Autodesk Inventor part; units mm, degrees
ref_plane "YZ Plane" through (0, 0, 0) normal (1, 0, 0) x (0, 1, 0)
ref_plane "XZ Plane" through (0, 0, 0) normal (0, 1, 0) x (-1, 0, 0)
ref_plane "XY Plane" through (0, 0, 0) normal (0, 0, 1) x (1, 0, 0)
sketch "Sketch1" plane through (0, 0, 0) normal (0, 1, 0) x (-1, 0, 0)
  line L0 (-4.5005, -6.5) -> (-3.283, -6.5)
  line L1 (-3.283, -6.5) -> (-2.9693, -6.948)
  line L2 (-2.9693, -6.948) -> (-2.9693, -8.2299)
  line L3 (-2.9693, -8.2299) -> (-2.0718, -8.2299)
  line L4 (-2.0718, -8.2299) -> (-2.0718, -7.0351)
  line L5 (-2.0718, -7.0351) -> (-1.8086, -6.5)
  line L6 (-1.8086, -6.5) -> (-0.6909, -6.5)
  line L7 (-0.6909, -6.5) -> (-0.4278, -7.0351)
  line L8 (-0.4278, -7.0351) -> (-0.4278, -8.2299)
  line L9 (-0.4278, -8.2299) -> (0.4698, -8.2299)
  line L10 (0.4698, -8.2299) -> (0.4698, -6.948)
  line L11 (0.4698, -6.948) -> (0.7835, -6.5)
  line L12 (0.7835, -6.5) -> (1.8077, -6.5)
  line L13 (1.8077, -6.5) -> (2.0708, -7.0351)
  line L14 (2.0708, -7.0351) -> (2.0708, -8.2299)
  line L15 (2.0708, -8.2299) -> (2.9683, -8.2299)
  line L16 (2.9683, -8.2299) -> (2.9683, -6.948)
  line L17 (2.9683, -6.948) -> (3.2821, -6.5)
  line L18 (3.2821, -6.5) -> (4.4995, -6.5)
  line L19 (4.4995, -6.5) -> (5.4995, -5.5)
  line L20 (5.4995, -5.5) -> (5.4995, 1.9247)
  line L21 (5.4995, 1.9247) -> (2.4995, 5.5)
  line L22 (2.4995, 5.5) -> (0.4698, 5.5)
  line L23 (0.4698, 5.5) -> (0.4698, 6.6191)
  line L24 (0.4698, 6.6191) -> (-0.4278, 6.6191)
  line L25 (-0.4278, 6.6191) -> (-0.4278, 5.5)
  line L26 (-0.4278, 5.5) -> (-2.5005, 5.5)
  line L27 (-2.5005, 5.5) -> (-5.5005, 1.9247)
  line L28 (-5.5005, 1.9247) -> (-5.5005, -5.5)
  line L29 (-5.5005, -5.5) -> (-4.5005, -6.5)
  circle A0 centre (-0.0005, -2.3274) radius 0.7145
  line L30 (6.998, 7.6726) -> (-7.002, 7.6726)
  line L31 (-7.002, 7.6726) -> (-7.002, -17.3274)
  line L32 (-7.002, -17.3274) -> (6.998, -17.3274)
  line L33 (6.998, -17.3274) -> (6.998, 7.6726)
  circle A1 centre (-0.0005, -2.3274) radius 2.75
  line L34 (-0.002, -21.2436) -> (-0.002, 13.4129) construction
  point P0 (-0.002, -0.846)
  dimension "d0" = 14
  dimension "d1" = 25
  dimension "d2" = 5.5
  dimension "d19" = 7
  dimension "d22" = 10
extrude "Extrusion1" add sketch "Sketch1" along normal blind 1.6 contours L29 L28 L27 L26 L25 L24 L23 L22 L21 L20 L19 L18 L17 L16 L15 L14 L13 L12 L11 L10 L9 L8 L7 L6 L5 L4 L3 L2 L1 L0 | L33 L32 L31 L30
sketch "Sketch2" plane through (0, 1.6, 0) normal (0, 1, 0) x (1, 0, 0)
  line L0 (-6.998, 17.3274) -> (-6.998, -7.6726)
  line L1 (7.002, 17.3274) -> (-6.998, 17.3274)
  line L2 (-6.998, -7.6726) -> (7.002, -7.6726)
  line L3 (7.002, -7.6726) -> (7.002, 17.3274)
  line L4 (7.002, 17.3274) -> (-6.998, 17.3274)
  line L5 (-6.998, 17.3274) -> (-6.998, -7.6726)
  circle A0 centre (5.002, -4.6726) radius 0.8
  circle A1 centre (5.002, 11.3274) radius 0.8
  circle A2 centre (-4.998, 11.3274) radius 0.8
  circle A3 centre (-4.998, -4.6726) radius 0.8
  point P0 (0, 0)
  dimension "d5" = 1.6
  dimension "d6" = 1.6
  dimension "d7" = 1.6
  dimension "d8" = 1.6
  dimension "d9" = 2
  dimension "d10" = 3
  dimension "d11" = 3
  dimension "d12" = 2
  dimension "d13" = 2
  dimension "d15" = 2
  dimension "d20" = 16
  dimension "d21" = 16
extrude "Extrusion2" cut sketch "Sketch2" against normal blind 1.6 contours A0 | A1 | A2 | A3
fillet "Fillet1" radius 2 4 edges at (-6.998, 0.8, 7.6726) (7.002, 0.8, 7.6726) (-6.998, 0.8, -17.3274) (7.002, 0.8, -17.3274)
equation "\"d19\" = 0.5 * d0"
equation "\"d5\" = d7"
equation "\"d6\" = d7"
equation "\"d8\" = d7"
equation "\"d10\" = d11"
equation "\"d20\" = d21"
properties part number "potentiometerpcb"
Part model, mm, in its own coordinate system. Give positions to 0.01 mm unless a question says otherwise; leave off trailing zeros. Order: outer loops, then holes, each group sorted by start corner. A loop starts at its lowest first (then second) coordinate and runs counter-clockwise, first axis right, second up. Notation, with made-up numbers: (-20.75, 65) - (-6.75, 65) arc R11 ccw to (-6.75, 79) - close; hole circle Ø6 at (4, 83). An arc over 180 degrees is marked (long way). One line per question, with ' | ' between items.
1. Drill centre lines: probe 1 along Z at (x, y) = (5.5, 1.4); probe 2 along Z at (x, y) = (5.25, 0.85); probe 3 along X at (y, z) = (0.85, 4.25). Where is each one in solid material? Low to high.
Filled in:
probe 1: -17.26 to -11.95, -10.7 to 4.05, 5.3 to 7.61 | probe 2: -17.31 to -12.09, -10.57 to 3.91, 5.43 to 7.66 | probe 3: -7 to -5.68, -4.32 to 4.32, 5.68 to 7
2. Pull direction Z, two halves, no side cores. Call faces 1 (the face through (-6.998, 1, -5)), 2 (the face through (6.401, 0.811, 7.102)), 3 (the face through (-5.6, 0.8, -10.8)): +Z half, -Z half, draft (parallel to the pull), parting line (faces both ways), or undercut.
Filled in:
face 1: draft | face 2: +Z half | face 3: undercut
3. Band-saw the part on A-A on z = -4.5. List the corners of the cut face in (x, y), then the cut area to 3 significant figures.
Filled in:
outline: (-7, 0) - (-1.69, 0) - (-1.69, 1.6) - (-7, 1.6) - close; (1.69, 0) - (7, 0) - (7, 1.6) - (1.69, 1.6) - close | area: 17.0 mm²
4. Band-saw the part on C-C on x = 5.5. List the corners of the cut face in (y, z), then the cut area to 3 significant figures.
Filled in:
outline: (0, -17.26) - (1.6, -17.26) - (1.6, -11.95) - (0, -11.95) - close; (0, -10.7) - (1.6, -10.7) - (1.6, 4.05) - (0, 4.05) - close; (0, 5.3) - (1.6, 5.3) - (1.6, 7.61) - (0, 7.61) - close | area: 35.8 mm²
5. Band-saw the part on B-B on x = -0.25. List the corners of the cut face in (y, z), then the cut area to 3 significant figures.
Filled in:
outline: (0, -17.33) - (1.6, -17.33) - (1.6, -5.07) - (0, -5.07) - close; (0, 0.41) - (1.6, 0.41) - (1.6, 7.67) - (0, 7.67) - close | area: 31.2 mm²
6. Band-saw the part on D-D on y = 0.7. List the corners of the cut face in (x, z).
Filled in:
outline: (-7, -15.33) arc R2 ccw to (-5, -17.33) - (5, -17.33) arc R2 ccw to (7, -15.33) - (7, 5.67) arc R2 ccw to (5, 7.67) - (-5, 7.67) arc R2 ccw to (-7, 5.67) - close; hole circle Ø1.6 at (-5, -11.33); hole circle Ø1.6 at (-5, 4.67); hole circle Ø5.5 at (0, -2.33); hole circle Ø1.6 at (5, -11.33); hole circle Ø1.6 at (5, 4.67)
7. Drop a flat-ended pin along its axis: P1, Ø1, axis at x = 5, z = 4.67, coming from the -Y side. Give the stop position or say it passes through.
Filled in:
P1: through
